For this review, take the finished solid that the model builds, in its own axes (mm). Round coordinates to 2 decimals unless told otherwise and drop trailing zeros. Write each loop counter-clockwise with the first axis right and the second up, starting at its lowest first coordinate (ties: lowest second). Pieces come first, ordered by that corner, then holes. Notation, with made-up numbers: M 33,87.5 L 86,87.5 A14 cw 86,110.5 Z; hole C 37,15.5 d6. An arc over 180 degrees is marked long. One line per question, with ' | ' between items.
```python
from build123d import *

# Parameters (mm, degrees)
F0_R          = 25
F0_R_2        = 11.5
F1_DEPTH      = 17.5
F1_DEPTH_BACK = 17.5
F0_R_3        = 5
F2_DEPTH      = 6
F3_DEPTH      = 6
F4_R          = 8.4
F6_DEPTH      = 83.1


with BuildPart() as f1:
    # F0 (on Front) → F1 (new body, two sides)
    with BuildSketch(Plane.XZ) as f1_sk:
        Circle(F0_R)
        Circle(F0_R_2, mode=Mode.SUBTRACT)
    extrude(amount=F1_DEPTH)
    extrude(f1_sk.sketch, amount=-F1_DEPTH_BACK)

    # F0 (on Front) → F2 (join)
    with BuildSketch(Plane.XZ):
        Circle(F0_R_2)
        Circle(F0_R_3, mode=Mode.SUBTRACT)
    extrude(amount=F2_DEPTH)

    # F0 (on Front) → F3 (join)
    with BuildSketch(Plane.XZ):
        Circle(F0_R_2)
        Circle(F0_R_3, mode=Mode.SUBTRACT)
    extrude(amount=-F3_DEPTH)

    # F4
    f4_edges = [f1.edges().sort_by_distance(p)[0] for p in [
        (-25, -17.5, 0),
        (-25, 17.5, 0),
    ]]
    fillet(f4_edges, radius=F4_R)

    # F6 (intersect): a face of the model
    f6_faces = [f1.faces().sort_by_distance(p)[0] for p in [
        (-16.1304810973, 17.5, 0),
    ]]
    extrude(f6_faces, amount=-F6_DEPTH, mode=Mode.INTERSECT)


solid = f1.part
```
Item 1: Take a section at C-C (y = -7.5). Write out the cut boundary in (x, z), then the cut area to 3 significant figures.
Results:
outline: C 0,0 d33.2; hole C 0,0 d23 | area: 450 mm2
Item 2: To check wall thickness, follow line 1 along Z through (x, y) = (0, -7); line 2 along Z through (x, y) = (-1.5, 14.5); line 3 along X through (y, z) = (-7, 5.5). State the ranges of each line that lie inside material, in increasing order. Write a range as from..to.
Results:
line 1: -16.6..-11.5, 11.5..16.6 | line 2: -16.53..-11.4, 11.4..16.53 | line 3: -15.66..-10.1, 10.1..15.66
Item 3: Take a section at B-B (z = 0). Write out the cut boundary in (x, y).
Results:
outline: M -16.6,-17.5 L -11.5,-17.5 L -11.5,17.5 L -16.6,17.5 Z; M 11.5,-17.5 L 16.6,-17.5 L 16.6,17.5 L 11.5,17.5 Z
Item 4: Mouldability with a two-part tool opening along X and no side actions: class faces 1 (the face through (-4, -17.5, -11)), 2 (the face through (-3.599, 0.245, -16.205)), 3 (the face through (-1.5, -0.2, 11.4)) as +X half, -X half, draft (parallel to the pull), parting line (faces both ways), or undercut.
Results:
face 1: draft | face 2: parting line | face 3: undercut
Item 5: Take a section at A-A (x = 0). Write out the cut boundary in (y, z).
Results:
outline: M -17.5,-16.6 L 17.5,-16.6 L 17.5,-11.5 L -17.5,-11.5 Z; M -17.5,11.5 L 17.5,11.5 L 17.5,16.6 L -17.5,16.6 Z
Item 6: Insertion check: pin 1 Ø1.5 at (x, z) = (-5.5, -10) entering from +Y; pin 2 Ø2 at (x, y) = (4.5, 8.5) entering from -Z; pin 3 Ø2 at (x, y) = (2.5, 0.5) entering from +Z. Each pin has a flat end and moves straight along its axis. Give the tip position at first contact, or say it passes through.
Results:
pin 1: y = 17.5 | pin 2: z = -16.23 | pin 3: z = 16.53
Item 7: Take a section at D-D (z = 12). Write out the cut boundary in (x, y).
Results:
outline: M -11.47,-17.5 L 11.47,-17.5 L 11.47,17.5 L -11.47,17.5 Z
